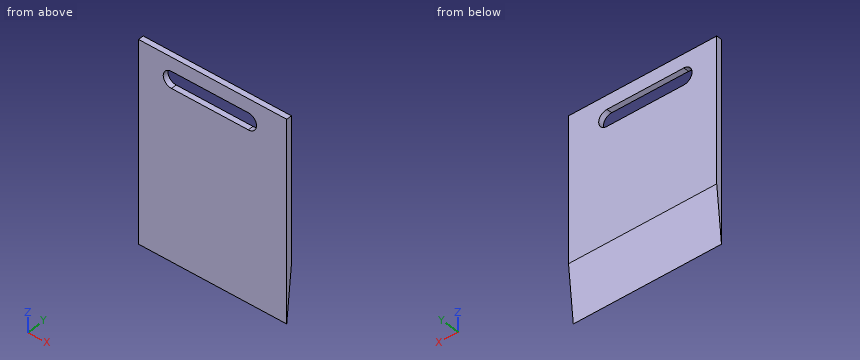
```python
from build123d import *

# Parameters (mm, degrees)
SALIENTE_EXTRUIR1_DEPTH = 13.5
CORTAR_EXTRUIR1_DEPTH   = 23.50555487


with BuildPart() as part:
    # Croquis1 → Saliente-Extruir1 (new body)
    with BuildSketch(Plane(origin=(0, 0, 0), x_dir=(0, 0, -1), z_dir=(1, 0, 0))):
        Polygon((0, 0), (18, 0), (13, 0.5), (0, 0.5), align=None)
    extrude(amount=SALIENTE_EXTRUIR1_DEPTH)

    # Croquis2 → Cortar-Extruir1 (cut, through all)
    with BuildSketch(Plane(origin=(0, 0.5, 0), x_dir=(1, 0, 0), z_dir=(0, 1, 0))):
        with BuildLine():
            Line((3, 2.75), (10, 2.75))
            ThreePointArc((10, 2.75), (10.75, 2), (10, 1.25))
            Line((10, 1.25), (3, 1.25))
            ThreePointArc((3, 1.25), (2.25, 2), (3, 2.75))
        make_face()
    extrude(amount=-CORTAR_EXTRUIR1_DEPTH, mode=Mode.SUBTRACT)


solid = part.part
```
The model under review builds one solid part; all positions refer to its coordinate system, in mm. Round coordinates to 2 decimals unless told otherwise and drop trailing zeros. Loops run counter-clockwise (first coordinate to the right, second up) from the corner with the lowest first, then second, coordinate; pieces in that order, holes last. Notation, with made-up numbers: M 38.5,29.5 L 97.5,29.5 A17 cw 97.5,55.5 Z; hole C 21,11 d6. An arc over 180 degrees is marked long. Write item = value, one per line.
Item 1: Take a section at A-A on x = 8.75. Write out the cut boundary in (y, z).
Return value:
outline = M 0,-18 L 0.5,-13 L 0.5,-2.75 L 0,-2.75 Z; M 0,-1.25 L 0.5,-1.25 L 0.5,0 L 0,0 Z
Item 2: Take a section at B-B on y = 0.15. Write out the cut boundary in (x, z), then the cut area to 3 significant figures.
Return value:
outline = M 0,-16.5 L 13.5,-16.5 L 13.5,0 L 0,0 Z; hole M 3,-2.75 L 10,-2.75 A0.75 ccw 10,-1.25 L 3,-1.25 A0.75 ccw Z
area = 210 mm2
Item 3: For line 1 (X direction, y = 0.4, z = -2.25); line 2 (Y direction, x = 4.5, z = -16); line 3 (Y direction, x = 6, z = -13.5), list the stretches that pass through material, from the lowest coordinate up. Write a range as [from, to].
Return value:
line_1 = [0, 2.29], [10.71, 13.5]
line_2 = [0, 0.2]
line_3 = [0, 0.45]
Item 4: Take a section at D-D on z = -16.5. Write out the cut boundary in (x, y).
Return value:
outline = M 0,0 L 13.5,0 L 13.5,0.15 L 0,0.15 Z
Item 5: Take a section at C-C on z = -2. Write out the cut boundary in (x, y).
Return value:
outline = M 0,0 L 2.25,0 L 2.25,0.5 L 0,0.5 Z; M 10.75,0 L 13.5,0 L 13.5,0.5 L 10.75,0.5 Z
